CAD build for the part. Positions are in the model's coordinates, mm. A direction names the side the tool comes from. Give positions to 0.01 mm unless a question says otherwise; leave off trailing zeros. Loops run counter-clockwise (first coordinate to the right, second up) from the corner with the lowest first, then second, coordinate; pieces in that order, holes last. Notation, with made-up numbers: M 13,49 L 46,49 A25 ccw 46,75 Z; hole C 47.25,-27 d4. An arc over 180 degrees is marked long. One line per question, with ' | ' between items.
```python
from build123d import *

# Parameters (mm, degrees)
SKETCH2_W                = 110
SKETCH2_H                = 110
SKETCH2_W_2              = 100
SKETCH2_H_2              = 100
BOSS_EXTRUDE1_DEPTH      = 89
SKETCH3_W                = 110
SKETCH3_H                = 110
BOSS_EXTRUDE2_DEPTH      = 8
CUT_EXTRUDE1_REACH       = 112
SKETCH6_W                = 60
SKETCH6_H                = 58
SKETCH9_W                = 110
SKETCH9_H                = 110
BOSS_EXTRUDE3_DEPTH      = 3
CUT_EXTRUDE2_REACH       = 63
SKETCH10_R               = 7.5
BOSS_EXTRUDE4_DEPTH      = 1.5
BOSS_EXTRUDE5_DEPTH      = 1.5
SKETCH14_R               = 3
CUT_EXTRUDE3_DEPTH       = 73
SKETCH15_W               = 2
SKETCH15_H               = 2
CUT_EXTRUDE4_DEPTH       = 113
CUT_EXTRUDE4_DEPTH_BACK  = 13
CUT_EXTRUDE5_REACH       = 63
SKETCH16_R               = 2.5
SKETCH17_R               = 14
SKETCH17_R_2             = 11
BOSS_EXTRUDE6_DEPTH      = 7
CUT_EXTRUDE8_REACH       = 7
SKETCH20_R               = 2
SKETCH18_R               = 2
CUT_EXTRUDE6_DEPTH       = 73.5
CUT_EXTRUDE7_REACH       = 63
SKETCH19_R               = 2
SKETCH21_R               = 24
SKETCH21_R_2             = 21
BOSS_EXTRUDE7_DEPTH      = 5
CUT_EXTRUDE9_REACH       = 46
SKETCH23_W               = 100
SKETCH23_H               = 100
SKETCH24_W               = 100
SKETCH24_H               = 100
BOSS_EXTRUDE8_DEPTH      = 20
SKETCH25_R               = 24
CUT_EXTRUDE10_DEPTH      = 10
CUT_EXTRUDE10_DEPTH_BACK = 26
SKETCH26_R               = 3
CUT_EXTRUDE11_DEPTH      = 26
M3_TAPPED_HOLE1_D        = 2.5
M3_TAPPED_HOLE1_DEPTH    = 6.748924226
M3_TAPPED_HOLE1_TIP      = 0.751075774
M3_TAPPED_HOLE2_D        = 2.5
M3_TAPPED_HOLE2_DEPTH    = 6.748924226
M3_TAPPED_HOLE2_TIP      = 0.751075774


with BuildPart() as part:
    # Sketch2 → Boss-Extrude1 (new body)
    with BuildSketch(Plane(origin=(0, 0, 0), x_dir=(1, 0, 0), z_dir=(0, 1, 0))):
        Rectangle(SKETCH2_W, SKETCH2_H)
        Rectangle(SKETCH2_W_2, SKETCH2_H_2, mode=Mode.SUBTRACT)
    extrude(amount=BOSS_EXTRUDE1_DEPTH)

    # Sketch3 → Boss-Extrude2 (add)
    with BuildSketch(Plane(origin=(0, 89, 0), x_dir=(1, 0, 0), z_dir=(0, 1, 0))):
        Rectangle(SKETCH3_W, SKETCH3_H)
    extrude(amount=BOSS_EXTRUDE2_DEPTH)

    # Sketch6 → Cut-Extrude1 (cut, up to next)
    with BuildSketch(Plane.XY.offset(55), mode=Mode.PRIVATE) as cut_extrude1_sk1:
        with Locations((0, 29)):
            Rectangle(SKETCH6_W, SKETCH6_H)
    cut_extrude1_tool1 = extrude(cut_extrude1_sk1.sketch, amount=-CUT_EXTRUDE1_REACH, mode=Mode.PRIVATE) & part.part
    add(cut_extrude1_tool1.solids().sort_by_distance((0, 29, 55))[0], mode=Mode.SUBTRACT)

    # Sketch8 → Cut-Revolve1 (revolve, cut)
    with BuildSketch(Plane.XY):
        Polygon((0, 97), (-21, 97), (-21, 92.5), (-16.2, 92.5), (-16.2, 88.5), (0, 88.5), align=None)
    revolve(axis=Axis((0, 0, 0), (0, 1, 0)), mode=Mode.SUBTRACT)

    # Sketch9 → Boss-Extrude3 (add)
    with BuildSketch(Plane.XZ.offset(-58)):
        Rectangle(SKETCH9_W, SKETCH9_H)
    extrude(amount=-BOSS_EXTRUDE3_DEPTH)

    # Sketch10 → Cut-Extrude2 (cut, up to next)
    with BuildSketch(Plane(origin=(0, 61, 0), x_dir=(1, 0, 0), z_dir=(0, 1, 0)), mode=Mode.PRIVATE) as cut_extrude2_sk1:
        Circle(SKETCH10_R)
    cut_extrude2_tool1 = extrude(cut_extrude2_sk1.sketch, amount=-CUT_EXTRUDE2_REACH, mode=Mode.PRIVATE) & part.part
    add(cut_extrude2_tool1.solids().sort_by_distance((0, 61, 0))[0], mode=Mode.SUBTRACT)

    # Sketch11 → Boss-Extrude4 (add, symmetric)
    with BuildSketch(Plane.XY):
        Polygon((-50, 89), (-35, 89), (-50, 69), align=None)
    boss_extrude4 = extrude(amount=BOSS_EXTRUDE4_DEPTH, both=True)

    # Mirror1: Boss-Extrude4 across plane
    add(boss_extrude4.mirror(Plane(origin=(0, 0, 0), x_dir=(0, 0, 1), z_dir=(1, 0, 0))))

    # Sketch12 → Boss-Extrude5 (add, symmetric)
    with BuildSketch(Plane(origin=(0, 0, 0), x_dir=(0, 0, -1), z_dir=(1, 0, 0))):
        Polygon((-35, 89), (-50, 89), (-50, 69), align=None)
    boss_extrude5 = extrude(amount=BOSS_EXTRUDE5_DEPTH, both=True)

    # Mirror2: Boss-Extrude5 across plane
    add(boss_extrude5.mirror(Plane.XY))

    # Sketch14 → Cut-Extrude3 (cut)
    with BuildSketch(Plane(origin=(0, 97, 0), x_dir=(1, 0, 0), z_dir=(0, 1, 0))):
        with Locations((40, 40)):
            Circle(SKETCH14_R)
        with Locations((-40, -40)):
            Circle(SKETCH14_R)
    extrude(amount=-CUT_EXTRUDE3_DEPTH, mode=Mode.SUBTRACT)

    # Sketch15 → Cut-Extrude4 (cut, two sides)
    with BuildSketch(Plane(origin=(-50, 0, 0), x_dir=(0, 0, -1), z_dir=(1, 0, 0))) as cut_extrude4_sk:
        with Locations((-24, 62)):
            Rectangle(SKETCH15_W, SKETCH15_H)
        with Locations((24, 62)):
            Rectangle(SKETCH15_W, SKETCH15_H)
    extrude(amount=CUT_EXTRUDE4_DEPTH, mode=Mode.SUBTRACT)
    extrude(cut_extrude4_sk.sketch, amount=-CUT_EXTRUDE4_DEPTH_BACK, mode=Mode.SUBTRACT)

    # Sketch16 → Cut-Extrude5 (cut, up to next)
    with BuildSketch(Plane(origin=(0, 61, 0), x_dir=(1, 0, 0), z_dir=(0, 1, 0)), mode=Mode.PRIVATE) as cut_extrude5_sk1:
        with Locations((-13.5, 13.5)):
            Circle(SKETCH16_R)
    cut_extrude5_tool1 = extrude(cut_extrude5_sk1.sketch, amount=-CUT_EXTRUDE5_REACH, mode=Mode.PRIVATE) & part.part
    add(cut_extrude5_tool1.solids().sort_by_distance((-13.5, 61, -13.5))[0], mode=Mode.SUBTRACT)
    # Sketch16 → Cut-Extrude5 (cut, up to next)
    with BuildSketch(Plane(origin=(0, 61, 0), x_dir=(1, 0, 0), z_dir=(0, 1, 0)), mode=Mode.PRIVATE) as cut_extrude5_sk2:
        with Locations((-13.5, -36)):
            Circle(SKETCH16_R)
    cut_extrude5_tool2 = extrude(cut_extrude5_sk2.sketch, amount=-CUT_EXTRUDE5_REACH, mode=Mode.PRIVATE) & part.part
    add(cut_extrude5_tool2.solids().sort_by_distance((-13.5, 61, 36))[0], mode=Mode.SUBTRACT)
    # Sketch16 → Cut-Extrude5 (cut, up to next)
    with BuildSketch(Plane(origin=(0, 61, 0), x_dir=(1, 0, 0), z_dir=(0, 1, 0)), mode=Mode.PRIVATE) as cut_extrude5_sk3:
        with Locations((13.5, -36)):
            Circle(SKETCH16_R)
    cut_extrude5_tool3 = extrude(cut_extrude5_sk3.sketch, amount=-CUT_EXTRUDE5_REACH, mode=Mode.PRIVATE) & part.part
    add(cut_extrude5_tool3.solids().sort_by_distance((13.5, 61, 36))[0], mode=Mode.SUBTRACT)
    # Sketch16 → Cut-Extrude5 (cut, up to next)
    with BuildSketch(Plane(origin=(0, 61, 0), x_dir=(1, 0, 0), z_dir=(0, 1, 0)), mode=Mode.PRIVATE) as cut_extrude5_sk4:
        with Locations((13.5, 13.5)):
            Circle(SKETCH16_R)
    cut_extrude5_tool4 = extrude(cut_extrude5_sk4.sketch, amount=-CUT_EXTRUDE5_REACH, mode=Mode.PRIVATE) & part.part
    add(cut_extrude5_tool4.solids().sort_by_distance((13.5, 61, -13.5))[0], mode=Mode.SUBTRACT)

    # Sketch17 → Boss-Extrude6 (add)
    with BuildSketch(Plane(origin=(0, 61, 0), x_dir=(1, 0, 0), z_dir=(0, 1, 0))):
        Circle(SKETCH17_R)
        Circle(SKETCH17_R_2, mode=Mode.SUBTRACT)
    extrude(amount=BOSS_EXTRUDE6_DEPTH)

    # Sketch20 → Cut-Extrude8 (cut, up to next)
    with BuildSketch(Plane.XY.offset(-50), mode=Mode.PRIVATE) as cut_extrude8_sk1:
        with Locations((10, 48)):
            Circle(SKETCH20_R)
    cut_extrude8_tool1 = extrude(cut_extrude8_sk1.sketch, amount=-CUT_EXTRUDE8_REACH, mode=Mode.PRIVATE) & part.part
    add(cut_extrude8_tool1.solids().sort_by_distance((10, 48, -50))[0], mode=Mode.SUBTRACT)
    # Sketch20 → Cut-Extrude8 (cut, up to next)
    with BuildSketch(Plane.XY.offset(-50), mode=Mode.PRIVATE) as cut_extrude8_sk2:
        with Locations((-10, 48)):
            Circle(SKETCH20_R)
    cut_extrude8_tool2 = extrude(cut_extrude8_sk2.sketch, amount=-CUT_EXTRUDE8_REACH, mode=Mode.PRIVATE) & part.part
    add(cut_extrude8_tool2.solids().sort_by_distance((-10, 48, -50))[0], mode=Mode.SUBTRACT)

    # Sketch18 → Cut-Extrude6 (cut, symmetric)
    with BuildSketch(Plane(origin=(0, 0, 0), x_dir=(0, 0, -1), z_dir=(1, 0, 0))):
        with Locations((10, 48)):
            Circle(SKETCH18_R)
        with Locations((-10, 48)):
            Circle(SKETCH18_R)
    extrude(amount=CUT_EXTRUDE6_DEPTH, both=True, mode=Mode.SUBTRACT)

    # Sketch19 → Cut-Extrude7 (cut, up to next)
    with BuildSketch(Plane(origin=(0, 61, 0), x_dir=(1, 0, 0), z_dir=(0, 1, 0)), mode=Mode.PRIVATE) as cut_extrude7_sk1:
        with Locations((40, 10)):
            Circle(SKETCH19_R)
    cut_extrude7_tool1 = extrude(cut_extrude7_sk1.sketch, amount=-CUT_EXTRUDE7_REACH, mode=Mode.PRIVATE) & part.part
    add(cut_extrude7_tool1.solids().sort_by_distance((40, 61, -10))[0], mode=Mode.SUBTRACT)
    # Sketch19 → Cut-Extrude7 (cut, up to next)
    with BuildSketch(Plane(origin=(0, 61, 0), x_dir=(1, 0, 0), z_dir=(0, 1, 0)), mode=Mode.PRIVATE) as cut_extrude7_sk2:
        with Locations((40, -10)):
            Circle(SKETCH19_R)
    cut_extrude7_tool2 = extrude(cut_extrude7_sk2.sketch, amount=-CUT_EXTRUDE7_REACH, mode=Mode.PRIVATE) & part.part
    add(cut_extrude7_tool2.solids().sort_by_distance((40, 61, 10))[0], mode=Mode.SUBTRACT)
    # Sketch19 → Cut-Extrude7 (cut, up to next)
    with BuildSketch(Plane(origin=(0, 61, 0), x_dir=(1, 0, 0), z_dir=(0, 1, 0)), mode=Mode.PRIVATE) as cut_extrude7_sk3:
        with Locations((-40, -10)):
            Circle(SKETCH19_R)
    cut_extrude7_tool3 = extrude(cut_extrude7_sk3.sketch, amount=-CUT_EXTRUDE7_REACH, mode=Mode.PRIVATE) & part.part
    add(cut_extrude7_tool3.solids().sort_by_distance((-40, 61, 10))[0], mode=Mode.SUBTRACT)
    # Sketch19 → Cut-Extrude7 (cut, up to next)
    with BuildSketch(Plane(origin=(0, 61, 0), x_dir=(1, 0, 0), z_dir=(0, 1, 0)), mode=Mode.PRIVATE) as cut_extrude7_sk4:
        with Locations((-40, 10)):
            Circle(SKETCH19_R)
    cut_extrude7_tool4 = extrude(cut_extrude7_sk4.sketch, amount=-CUT_EXTRUDE7_REACH, mode=Mode.PRIVATE) & part.part
    add(cut_extrude7_tool4.solids().sort_by_distance((-40, 61, -10))[0], mode=Mode.SUBTRACT)
    # Sketch19 → Cut-Extrude7 (cut, up to next)
    with BuildSketch(Plane(origin=(0, 61, 0), x_dir=(1, 0, 0), z_dir=(0, 1, 0)), mode=Mode.PRIVATE) as cut_extrude7_sk5:
        with Locations((10, 40)):
            Circle(SKETCH19_R)
    cut_extrude7_tool5 = extrude(cut_extrude7_sk5.sketch, amount=-CUT_EXTRUDE7_REACH, mode=Mode.PRIVATE) & part.part
    add(cut_extrude7_tool5.solids().sort_by_distance((10, 61, -40))[0], mode=Mode.SUBTRACT)
    # Sketch19 → Cut-Extrude7 (cut, up to next)
    with BuildSketch(Plane(origin=(0, 61, 0), x_dir=(1, 0, 0), z_dir=(0, 1, 0)), mode=Mode.PRIVATE) as cut_extrude7_sk6:
        with Locations((-10, 40)):
            Circle(SKETCH19_R)
    cut_extrude7_tool6 = extrude(cut_extrude7_sk6.sketch, amount=-CUT_EXTRUDE7_REACH, mode=Mode.PRIVATE) & part.part
    add(cut_extrude7_tool6.solids().sort_by_distance((-10, 61, -40))[0], mode=Mode.SUBTRACT)

    # Sketch21 → Boss-Extrude7 (add)
    with BuildSketch(Plane(origin=(0, 97, 0), x_dir=(1, 0, 0), z_dir=(0, 1, 0))):
        Circle(SKETCH21_R)
        Circle(SKETCH21_R_2, mode=Mode.SUBTRACT)
    extrude(amount=BOSS_EXTRUDE7_DEPTH)

    # Sketch23 → Cut-Extrude9 (cut, up to next)
    with BuildSketch(Plane.XZ.offset(-58), mode=Mode.PRIVATE) as cut_extrude9_sk1:
        Rectangle(SKETCH23_W, SKETCH23_H)
    cut_extrude9_tool1 = extrude(cut_extrude9_sk1.sketch, amount=-CUT_EXTRUDE9_REACH, mode=Mode.PRIVATE) & part.part
    add(cut_extrude9_tool1.solids().sort_by_distance((0, 58, 0))[0], mode=Mode.SUBTRACT)

    # Sketch24 → Boss-Extrude8 (add)
    with BuildSketch(Plane.XZ.offset(-89)):
        Rectangle(SKETCH24_W, SKETCH24_H)
    extrude(amount=BOSS_EXTRUDE8_DEPTH)

    # Sketch25 → Cut-Extrude10 (cut, two sides)
    with BuildSketch(Plane(origin=(0, 92.5, 0), x_dir=(1, 0, 0), z_dir=(0, 1, 0))) as cut_extrude10_sk:
        Circle(SKETCH25_R)
    extrude(amount=CUT_EXTRUDE10_DEPTH, mode=Mode.SUBTRACT)
    extrude(cut_extrude10_sk.sketch, amount=-CUT_EXTRUDE10_DEPTH_BACK, mode=Mode.SUBTRACT)

    # Sketch26 → Cut-Extrude11 (cut)
    with BuildSketch(Plane(origin=(0, 89, 0), x_dir=(1, 0, 0), z_dir=(0, 1, 0))):
        with Locations((-40, -40)):
            Circle(SKETCH26_R)
        with Locations((40, 40)):
            Circle(SKETCH26_R)
    extrude(amount=-CUT_EXTRUDE11_DEPTH, mode=Mode.SUBTRACT)

    # M3 Tapped Hole1
    with Locations(Plane(origin=(-29, 97, 0), x_dir=(0, 0, 1), z_dir=(0, 1, 0))):
        with Locations((0, 0), (29, 29), (0, 58), (-29, 29)):
            Hole(M3_TAPPED_HOLE1_D / 2, depth=M3_TAPPED_HOLE1_DEPTH)
            with Locations((0, 0, -(M3_TAPPED_HOLE1_DEPTH + M3_TAPPED_HOLE1_TIP / 2))):  # 118° drill point
                Cone(0, M3_TAPPED_HOLE1_D / 2, M3_TAPPED_HOLE1_TIP, mode=Mode.SUBTRACT)

    # M3 Tapped Hole2
    with Locations(Plane(origin=(0, 69, 0), x_dir=(-1, 0, 0), z_dir=(0, -1, 0))):
        with Locations((0, -29), (29, 0), (0, 29), (-29, 0)):
            Hole(M3_TAPPED_HOLE2_D / 2, depth=M3_TAPPED_HOLE2_DEPTH)
            with Locations((0, 0, -(M3_TAPPED_HOLE2_DEPTH + M3_TAPPED_HOLE2_TIP / 2))):  # 118° drill point
                Cone(0, M3_TAPPED_HOLE2_D / 2, M3_TAPPED_HOLE2_TIP, mode=Mode.SUBTRACT)


solid = part.part
```
Item 1: 3-axis set-ups, long thin cutter, end or side, ignore diameter. For faces 5 (the flat face through (-1, 48, -55)), 6 (the flat face through (0, 58, 53)), 7 (the flat face through (-1, 34, -50)): which of +Z, -Z, +X, -X, +Y, -Y reach the whole face in a straight line?
Conclusion:
face 5: -Z, +X, -X, +Y, -Y | face 6: +Z, -Y | face 7: -Y
Item 2: Mould opens along Y. For faces 1 (the flat face through (-23, 69, 12)), 2 (the cylindrical face through (53, 46, 10)), 3 (the flat face through (-30, 29, 53)), 4 (the cylindrical face through (-52.465, 46.226, -10.923)) say: pulls with the +Y half, pulls with the -Y half, needs draft (parallel to the pull), parting line crosses it, or undercut.
Conclusion:
face 1: pulls with the -Y half | face 2: undercut | face 3: needs draft | face 4: undercut
Item 3: Saw through at A-A on y = 59.5. Give the cut face in (x, z), and give its area (3 significant figures).
Conclusion:
outline: M -55,-55 L 55,-55 L 55,55 L -55,55 Z; hole M -50,-50 L 50,-50 L 50,50 L -50,50 Z | area: 2,100 mm²
Item 4: Drill centre lines: line 1 along Z through (x, y) = (-38, 42); line 2 along Z through (x, y) = (0, 94.25). Where is each one in solid material? Low to high. Write a range as [from, to].
Conclusion:
line 1: [-55, -50], [50, 55] | line 2: [-55, -30.25], [-27.75, -24], [24, 27.75], [30.25, 55]
Item 5: Drop flat-ended pins along their axis: P1, Ø6, axis at x = 36, z = 6, coming from the -Y side; P2, Ø3, axis at y = 48, z = 10, coming from the -X side. Give the stop position or say it passes through.
Conclusion:
P1: y = 69 | P2: through
Item 6: Saw through at B-B on z = -40. Give the cut face in (x, y).
Conclusion:
outline: M -55,0 L -50,0 L -50,69 L 37,69 L 37,97 L -55,97 Z; M 43,69 L 50,69 L 50,0 L 55,0 L 55,97 L 43,97 Z
Item 7: Saw through at C-C on y = 79.5. Give the cut face in (x, z), and give its area (3 significant figures).
Conclusion:
outline: M -55,-55 L 55,-55 L 55,55 L -55,55 Z; hole C -40,40 d6; hole C 0,0 d48; hole C 40,-40 d6 | area: 10,200 mm²
Item 8: Saw through at D-D on x = 40. Give the cut face in (y, z), and give its area (3 significant figures).
Conclusion:
outline: M 0,-55 L 97,-55 L 97,-43 L 69,-43 L 69,-50 L 0,-50 Z; M 0,50 L 69,50 L 69,-37 L 97,-37 L 97,55 L 0,55 Z | area: 3,600 mm²
